Design review of the part built by this model. Coordinates are the model's own, in mm. A direction names the side the tool comes from. Coordinates: 2 decimals unless noted, no trailing zeros. Write each loop counter-clockwise with the first axis right and the second up, starting at its lowest first coordinate (ties: lowest second). Pieces come first, ordered by that corner, then holes.
Q1. Add section B-B, the plane y = 1. Give the boundary of the cut face in (x, z), plus the area to 3 significant figures.
Q2. Machinability: for faces 1 (the face through (12, 3, 20)), 2 (the face through (-21.68, 8.73, -24.55)), 3 (the face through (20, 7, 30)), 4 (the face through (21.72, 8.73, -24.62)), 5 (the face through (10.42, 8.73, -31.05)), which of the approach directions +Z, -Z, +X, -X, +Y, -Y give a long, thin tool a straight path to every point of the face, cutting with its end or side? Answer none if there is none.
Q3. Add section A-A, the plane z = 0. Give the boundary of the cut face in (x, y), plus the area to 3 significant figures.
Q4. The part is to be moulded in two halves that separate along X. For faces 6 (the face through (-10.42, 8.73, 31.05)), 7 (the face through (-32, 9, 6.5)), 8 (the face through (21.68, 8.73, 24.55)), say which applies: +X half, -X half, draft (parallel to the pull), parting line (faces both ways), or undercut.
Q5. Add section C-C, the plane x = 0. Give the boundary of the cut face in (y, z), plus the area to 3 significant figures.
Q6. Clearance check with flat-ended pins moving along their axes: pin 1 Ø3.5 at (x, z) = (-34, 2.5) entering from -Y; pin 2 Ø8 at (x, z) = (-1.5, -23) entering from +Y; pin 3 Ø2 at (y, z) = (1.5, -8) entering from +X; pin 4 Ø1.8 at (x, y) = (-32, 8.5) entering from +Z. State where each tip first meets the part, or that it passes through.
Q7. Add section D-D, the plane x = -17.5. Give the boundary of the cut face in (y, z), plus the area to 3 significant figures.
Q8. To check wall thickness, follow probe 1 along X at (y, z) = (9.55, 0); probe 2 along Z at (x, y) = (0.5, 4.5); probe 3 along Z at (x, y) = (-21.5, 8.5). State the ranges of each line that lie inside material, in increasing order.
from build123d import *

# Parameters (mm, degrees)
SKETCH1_R           = 26
SKETCH1_R_2         = 2.15
BOSS_EXTRUDE1_DEPTH = 10.5
SKETCH2_R           = 27.448916739
SKETCH2_R_2         = 22.85
BOSS_EXTRUDE2_DEPTH = 3
SKETCH3_R           = 44.09476296
SKETCH3_R_2         = 30
CUT_EXTRUDE1_DEPTH  = 7
SKETCH4_R           = 26.5
CUT_EXTRUDE2_DEPTH  = 7.5


with BuildPart() as part:
    # Sketch1 → Boss-Extrude1 (new body)
    with BuildSketch(Plane(origin=(0, 0, 0), x_dir=(1, 0, 0), z_dir=(0, 1, 0))):
        with BuildLine():
            Line((11.870834875, -33.560889132), (9.014519521, -28.613605816))
            ThreePointArc((9.014519521, -28.613605816), (0, -30), (-9.014519521, -28.613605816))
            Line((-9.014519521, -28.613605816), (-11.870834875, -33.560889132))
            ThreePointArc((-11.870834875, -33.560889132), (-20.75, -35.940054257), (-23.129165125, -27.060889132))
            Line((-23.129165125, -27.060889132), (-20.27284977, -22.113605816))
            ThreePointArc((-20.27284977, -22.113605816), (-25.980762114, -15), (-29.287369291, -6.5))
            Line((-29.287369291, -6.5), (-35, -6.5))
            ThreePointArc((-35, -6.5), (-41.5, 0), (-35, 6.5))
            Line((-35, 6.5), (-29.287369291, 6.5))
            ThreePointArc((-29.287369291, 6.5), (-25.980762114, 15), (-20.27284977, 22.113605816))
            Line((-20.27284977, 22.113605816), (-23.129165125, 27.060889132))
            ThreePointArc((-23.129165125, 27.060889132), (-20.75, 35.940054257), (-11.870834875, 33.560889132))
            Line((-11.870834875, 33.560889132), (-9.014519521, 28.613605816))
            ThreePointArc((-9.014519521, 28.613605816), (0, 30), (9.014519521, 28.613605816))
            Line((9.014519521, 28.613605816), (11.870834875, 33.560889132))
            ThreePointArc((11.870834875, 33.560889132), (20.75, 35.940054257), (23.129165125, 27.060889132))
            Line((23.129165125, 27.060889132), (20.27284977, 22.113605816))
            ThreePointArc((20.27284977, 22.113605816), (25.980762114, 15), (29.287369291, 6.5))
            Line((29.287369291, 6.5), (35, 6.5))
            ThreePointArc((35, 6.5), (41.5, 0), (35, -6.5))
            Line((35, -6.5), (29.287369291, -6.5))
            ThreePointArc((29.287369291, -6.5), (25.980762114, -15), (20.27284977, -22.113605816))
            Line((20.27284977, -22.113605816), (23.129165125, -27.060889132))
            ThreePointArc((23.129165125, -27.060889132), (20.75, -35.940054257), (11.870834875, -33.560889132))
        make_face()
        Circle(SKETCH1_R, mode=Mode.SUBTRACT)
        with Locations((35, 0)):
            Circle(SKETCH1_R_2, mode=Mode.SUBTRACT)
        with Locations((17.5, -30.310889132)):
            Circle(SKETCH1_R_2, mode=Mode.SUBTRACT)
        with Locations((-17.5, -30.310889132)):
            Circle(SKETCH1_R_2, mode=Mode.SUBTRACT)
        with Locations((-35, 0)):
            Circle(SKETCH1_R_2, mode=Mode.SUBTRACT)
        with Locations((-17.5, 30.310889132)):
            Circle(SKETCH1_R_2, mode=Mode.SUBTRACT)
        with Locations((17.5, 30.310889132)):
            Circle(SKETCH1_R_2, mode=Mode.SUBTRACT)
    extrude(amount=BOSS_EXTRUDE1_DEPTH)

    # Sketch2 → Boss-Extrude2 (add)
    with BuildSketch(Plane.XZ):
        Circle(SKETCH2_R)
        Circle(SKETCH2_R_2, mode=Mode.SUBTRACT)
    extrude(amount=-BOSS_EXTRUDE2_DEPTH)

    # Sketch3 → Cut-Extrude1 (cut)
    with BuildSketch(Plane.XZ):
        Circle(SKETCH3_R)
        Circle(SKETCH3_R_2, mode=Mode.SUBTRACT)
    extrude(amount=-CUT_EXTRUDE1_DEPTH, mode=Mode.SUBTRACT)

    # Sketch4 → Cut-Extrude2 (cut)
    with BuildSketch(Plane(origin=(0, 10.5, 0), x_dir=(1, 0, 0), z_dir=(0, 1, 0))):
        Circle(SKETCH4_R)
    extrude(amount=-CUT_EXTRUDE2_DEPTH, mode=Mode.SUBTRACT)


solid = part.part
Here are the results:
1. outline: circle Ø60 at (0, 0); hole circle Ø45.7 at (0, 0)
1. area: 1,190 mm2
2. face 1: +Y
2. face 2: -X, +Y, -Y
2. face 3: +Z, +X, -Y
2. face 4: +X, +Y, -Y
2. face 5: -Z, +Y, -Y
3. outline: (-41.5, 7) - (-37.15, 7) - (-37.15, 10.5) - (-41.5, 10.5) - close; (-32.85, 7) - (-30, 7) - (-30, 0) - (-22.85, 0) - (-22.85, 3) - (-26.5, 3) - (-26.5, 10.5) - (-32.85, 10.5) - close; (22.85, 0) - (30, 0) - (30, 7) - (32.85, 7) - (32.85, 10.5) - (26.5, 10.5) - (26.5, 3) - (22.85, 3) - close; (37.15, 7) - (41.5, 7) - (41.5, 10.5) - (37.15, 10.5) - close
3. area: 146 mm2
4. face 6: undercut
4. face 7: draft
4. face 8: +X half
5. outline: (0, -30) - (10.5, -30) - (10.5, -26.5) - (3, -26.5) - (3, -22.85) - (0, -22.85) - close; (0, 22.85) - (3, 22.85) - (3, 26.5) - (10.5, 26.5) - (10.5, 30) - (0, 30) - close
5. area: 95.4 mm2
6. pin 1: stops at y = 7
6. pin 2: stops at y = 10.5
6. pin 3: stops at x = 29.17
6. pin 4: stops at z = 6.5
7. outline: (0, -24.37) - (7, -24.37) - (7, -28.16) - (10.5, -28.16) - (10.5, -19.9) - (3, -19.9) - (3, -14.69) - (0, -14.69) - close; (0, 14.69) - (3, 14.69) - (3, 19.9) - (10.5, 19.9) - (10.5, 28.16) - (7, 28.16) - (7, 24.37) - (0, 24.37) - close; (7, -36.81) - (10.5, -36.81) - (10.5, -32.46) - (7, -32.46) - close; (7, 32.46) - (10.5, 32.46) - (10.5, 36.81) - (7, 36.81) - close
7. area: 182 mm2
8. probe 1: x = -41.5 to -37.15, -32.85 to -26.5, 26.5 to 32.85, 37.15 to 41.5
8. probe 2: z = -30 to -26.5, 26.5 to 30
8. probe 3: z = -35.43 to -24.24, -20.92 to -15.49, 15.49 to 20.92, 24.24 to 35.43
